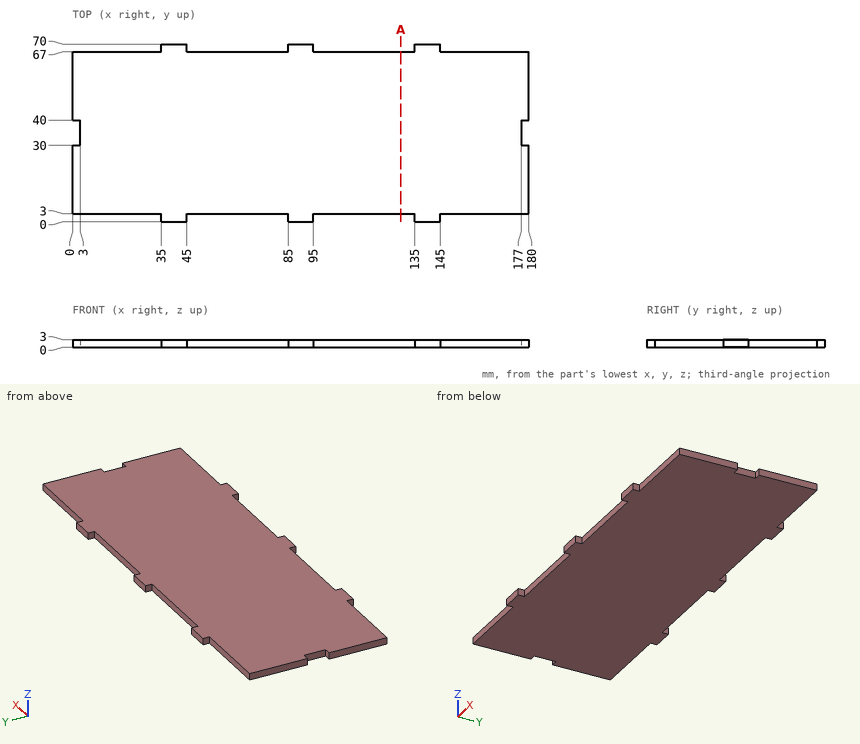
The figure shows three views and two pictorial views of one solid part (mm, origin at its lowest corner). Answer the questions. Give positions to 0.01 mm unless a question says otherwise; leave off trailing zeros. Order: outer loops, then holes, each group sorted by start corner. A loop starts at its lowest first (then second) coordinate and runs counter-clockwise, first axis right, second up. Notation, with made-up numbers: (-4.5, 21) -> (39.5, 21) arc R24 ccw to (39.5, 46) -> close; hole circle Ø4 at (45.25, 79). An arc over 180 degrees is marked (long way). Answer as CSV lines item,"result". Start each with the question number.
Q1. A cutting plane is placed at A-A (x = 129.5). Determine the outline of the cut face in (y, z), then the cut area to 3 significant figures.
Q2. Given pin 1 (1.5 mm diameter, centred on y = 35, z = 1, fed in from +X); pin 2 (1 mm diameter, centred on x = 122, z = 2, fed in from +Y); pin 3 (1.5 mm diameter, centred on y = 2, z = 1, fed in from -X); pin 4 (4 mm diameter, centred on x = 145.5, y = 33.5, fed in from -Z), each flat-ended and moving along its own axis, determine where each tip first touches the part or whether it passes through.
Q3. Find the intervals of material crossed by L1, parallel to Y at x = 123, z = 2; L2, parallel to X at y = 30.5, z = 2.75, in increasing order.
Results found:
1,outline,"(3, 0) -> (67, 0) -> (67, 3) -> (3, 3) -> close"
1,area,"192 mm2"
2,pin 1,"x = 177"
2,pin 2,"y = 67"
2,pin 3,"x = 35"
2,pin 4,"z = 0"
3,L1,"3 to 67"
3,L2,"3 to 177"
